```python
from build123d import *

# Parameters (mm, degrees)
F_01_START                                = 13
F_01_TPU_16_BY_5_GAUGE_DEPTH              = 61.40149944
F_02_CORD_END_BLOCK_DEPTH                 = 13
F_03_START                                = -0.2
S03_OPEN_TWO_EAR_PIN_CLEVIS_W             = 18
S03_OPEN_TWO_EAR_PIN_CLEVIS_H             = 4.5
F_03_OPEN_TWO_EAR_PIN_CLEVIS_DEPTH        = 11.8
F_04_START                                = -5.2
S04_SHOULDER_PIN_THROUGH_BOTH_EARS_R      = 2.08
F_04_SHOULDER_PIN_THROUGH_BOTH_EARS_DEPTH = 10.4


# Read off the part's stored shape, not the designer's step: 01 - TPU 16 by 5 gauge
with BuildPart() as part:
    # 01 - TPU 16 by 5 gauge outline → 01 - TPU 16 by 5 gauge (new body)
    with BuildSketch(Plane.XY.offset(F_01_START)):
        with BuildLine():
            ThreePointArc((-8, -4), (-7.707106781, -4.707106781), (-7, -5))
            Line((-7, -5), (7, -5))
            ThreePointArc((7, -5), (7.707106781, -4.707106781), (8, -4))
            Line((8, -4), (8, -1))
            ThreePointArc((8, -1), (7.707106781, -0.292893219), (7, 0))
            Line((7, 0), (-7, 0))
            ThreePointArc((-7, 0), (-7.707106781, -0.292893219), (-8, -1))
            Line((-8, -1), (-8, -4))
        make_face()
    extrude(amount=F_01_TPU_16_BY_5_GAUGE_DEPTH)

    # S02 - Cord end block → 02 - Cord end block (add)
    with BuildSketch(Plane.XY):
        with BuildLine():
            Line((-6, -5), (6, -5))
            ThreePointArc((6, -5), (7.414213562, -4.414213562), (8, -3))
            Line((8, -3), (8, 3))
            ThreePointArc((8, 3), (7.414213562, 4.414213562), (6, 5))
            Line((6, 5), (-6, 5))
            ThreePointArc((-6, 5), (-7.414213562, 4.414213562), (-8, 3))
            Line((-8, 3), (-8, -3))
            ThreePointArc((-8, -3), (-7.414213562, -4.414213562), (-6, -5))
        make_face()
    extrude(amount=F_02_CORD_END_BLOCK_DEPTH)

    # S03 - Open two-ear pin clevis → 03 - Open two-ear pin clevis (cut)
    with BuildSketch(Plane.XY.offset(F_03_START)):
        Rectangle(S03_OPEN_TWO_EAR_PIN_CLEVIS_W, S03_OPEN_TWO_EAR_PIN_CLEVIS_H)
    extrude(amount=F_03_OPEN_TWO_EAR_PIN_CLEVIS_DEPTH, mode=Mode.SUBTRACT)

    # S04 - Shoulder pin through both ears → 04 - Shoulder pin through both ears (cut)
    with BuildSketch(Plane(origin=(0, 0, 0), x_dir=(1, 0, 0), z_dir=(0, 1, 0)).offset(F_04_START)):
        with Locations(Location((-3.6, -6, 0), (0, 0, 90))):
            Circle(S04_SHOULDER_PIN_THROUGH_BOTH_EARS_R)
    extrude(amount=F_04_SHOULDER_PIN_THROUGH_BOTH_EARS_DEPTH, mode=Mode.SUBTRACT)


solid = part.part
```
Check sheet for the modelled part. Datum: model origin and axes. Units: mm. A direction names the side the tool comes from. Coordinates: 2 decimals unless noted, no trailing zeros. Write each loop counter-clockwise with the first axis right and the second up, starting at its lowest first coordinate (ties: lowest second). Pieces come first, ordered by that corner, then holes. Notation, with made-up numbers: M 35.25,-23 L 83.25,-23 A24 ccw 83.25,-1 Z; hole C 26,-14.75 d1. An arc over 180 degrees is marked long. Use one line per item in the form item = value.
Item 1: Gauge pin test, flat ends, axial feed: pin 1 Ø3 at (x, z) = (6, 26.5) entering from +Y; pin 2 Ø3 at (x, y) = (1.5, 3) entering from +Z. Record the tip position at first contact, or that the pin passes through.
Answer below:
pin_1 = 0
pin_2 = 13
Item 2: Sectioned sample at B-B, the plane x = -3.6. Record the cut outline in (y, z), and give its area (3 significant figures).
Answer below:
outline = M -5,0 L -2.25,0 L -2.25,3.92 L -5,3.92 Z; M -5,8.08 L -2.25,8.08 L -2.25,11.6 L 2.25,11.6 L 2.25,8.08 L 5,8.08 L 5,13 L 0,13 L 0,74.4 L -5,74.4 Z; M 2.25,0 L 5,0 L 5,3.92 L 2.25,3.92 Z
area = 362 mm^2
Item 3: Material ranges on L1, parallel to Y at x = -5.5, z = 9.5; L2, parallel to Z at x = 1.75, y = 4; L3, parallel to Z at x = 2.75, y = 0.75, recorded low to high. Write a range as from..to.
Answer below:
L1 = -5..-2.25, 2.25..5
L2 = 0..13
L3 = 11.6..13
Item 4: Release check for a two-part mould opening along Y. For faces 5 (the face through (7.5, -4.6, 13)), 6 (the face through (0, 0, 11.6)), 7 (the face through (0, 0, 43)) record: pulls with the +Y half, pulls with the -Y half, needs draft (parallel to the pull), parting line crosses it, or undercut.
Answer below:
face_5 = needs draft
face_6 = undercut
face_7 = pulls with the +Y half
Item 5: Sectioned sample at A-A, the plane z = 6. Record the cut outline in (x, y), and give its area (3 significant figures).
Answer below:
outline = M -8,-3 A2 ccw -6,-5 L -5.68,-5 L -5.68,-2.25 L -8,-2.25 Z; M -8,2.25 L -5.68,2.25 L -5.68,5 L -6,5 A2 ccw -8,3 Z; M -1.52,-5 L 6,-5 A2 ccw 8,-3 L 8,-2.25 L -1.52,-2.25 Z; M -1.52,2.25 L 8,2.25 L 8,3 A2 ccw 6,5 L -1.52,5 Z
area = 61.7 mm^2
Item 6: Sectioned sample at D-D, the plane x = -0.5. Record the cut outline in (y, z), and give its area (3 significant figures).
Answer below:
outline = M -5,0 L -2.25,0 L -2.25,11.6 L 2.25,11.6 L 2.25,0 L 5,0 L 5,13 L 0,13 L 0,74.4 L -5,74.4 Z
area = 385 mm^2
Item 7: Sectioned sample at C-C, the plane z = 44. Record the cut outline in (x, y).
Answer below:
outline = M -8,-4 A1 ccw -7,-5 L 7,-5 A1 ccw 8,-4 L 8,-1 A1 ccw 7,0 L -7,0 A1 ccw -8,-1 Z
Item 8: Set-up check for faces 1 (the face through (0, 5, 6)), 2 (the face through (7.4, -4.43, 6.41)), 3 (the face through (0, -2.25, 6)), 4 (the face through (-7.6, -4.44, 13)): record each of +Z, -Z, +X, -X, +Y, -Y from which the full face is reachable in a straight line by a thin tool's end or side.
Answer below:
face_1 = +Z, -Z, +X, -X, +Y
face_2 = -Z, +X, -Y
face_3 = -Z, +X, -X
face_4 = -Z, -X, -Y
